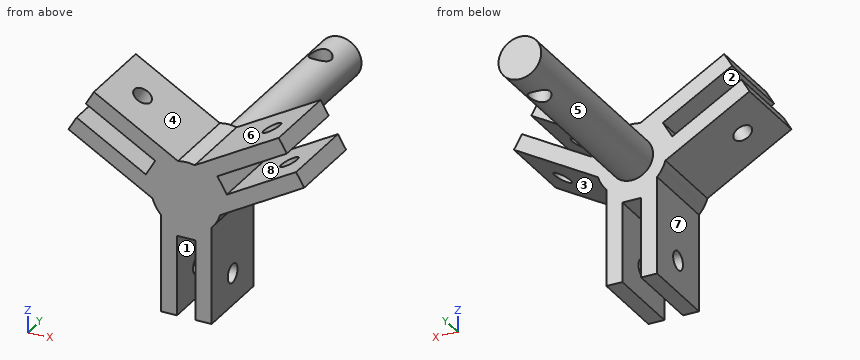
```python
from build123d import *

# Parameters (mm, degrees)
EXTRUDE_1_DEPTH     = 15
SKETCH_2_R          = 4
EXTRUDE_2_DEPTH     = 40
SKETCH_3_R          = 1.75
CUT_EXTRUDE_1_DEPTH = 15
SKETCH_4_R          = 1.75
CUT_EXTRUDE_2_DEPTH = 15
SKETCH_5_R          = 1.75
CUT_EXTRUDE_3_DEPTH = 15
SKETCH_7_R          = 2
CUT_EXTRUDE_4_DEPTH = 15


with BuildPart() as part:
    # 草圖1 → 填料-伸長1 (new body)
    with BuildSketch(Plane(origin=(0, 0, 0), x_dir=(1, 0, 0), z_dir=(0, 1, 0))):
        with BuildLine():
            Line((6.314953067, 1.838887704), (22.070508076, -7.257586221))
            Line((22.070508076, -7.257586221), (20.570508076, -9.855662433))
            Line((20.570508076, -9.855662433), (7.580127019, -2.355662433))
            Line((7.580127019, -2.355662433), (5.830127019, -5.386751346))
            Line((5.830127019, -5.386751346), (18.820508076, -12.886751346))
            Line((18.820508076, -12.886751346), (17.320508076, -15.484827557))
            Line((17.320508076, -15.484827557), (1.564953067, -6.388353632))
            ThreePointArc((1.564953067, -6.388353632), (0, -6.577244121), (-1.564953067, -6.388353632))
            Line((-1.564953067, -6.388353632), (-17.320508076, -15.484827557))
            Line((-17.320508076, -15.484827557), (-18.820508076, -12.886751346))
            Line((-18.820508076, -12.886751346), (-5.830127019, -5.386751346))
            Line((-5.830127019, -5.386751346), (-7.580127019, -2.355662433))
            Line((-7.580127019, -2.355662433), (-20.570508076, -9.855662433))
            Line((-20.570508076, -9.855662433), (-22.070508076, -7.257586221))
            Line((-22.070508076, -7.257586221), (-6.314953067, 1.838887704))
            ThreePointArc((-6.314953067, 1.838887704), (-5.696060496, 3.28862206), (-4.75, 4.549465928))
            Line((-4.75, 4.549465928), (-4.75, 22.742413779))
            Line((-4.75, 22.742413779), (-1.75, 22.742413779))
            Line((-1.75, 22.742413779), (-1.75, 7.742413779))
            Line((-1.75, 7.742413779), (1.75, 7.742413779))
            Line((1.75, 7.742413779), (1.75, 22.742413779))
            Line((1.75, 22.742413779), (4.75, 22.742413779))
            Line((4.75, 22.742413779), (4.75, 4.549465928))
            ThreePointArc((4.75, 4.549465928), (5.696060496, 3.28862206), (6.314953067, 1.838887704))
        make_face()
    extrude(amount=EXTRUDE_1_DEPTH)

    # 草圖2 → 填料-伸長2 (add)
    with BuildSketch(Plane(origin=(0, 15, 0), x_dir=(1, 0, 0), z_dir=(0, 1, 0))):
        Circle(SKETCH_2_R)
    extrude(amount=EXTRUDE_2_DEPTH)

    # 草圖3 → 除料-伸長1 (cut)
    with BuildSketch(Plane(origin=(4.75, 0, 0), x_dir=(0, 0, -1), z_dir=(1, 0, 0))):
        with Locations((16.742413779, 7.5)):
            Circle(SKETCH_3_R)
    extrude(amount=-CUT_EXTRUDE_1_DEPTH, mode=Mode.SUBTRACT)

    # 草圖4 → 除料-伸長2 (cut)
    with BuildSketch(Plane(origin=(-2.375, 0, -4.113620668), x_dir=(-0.866025404, 0, 0.5), z_dir=(-0.5, 0, -0.866025404))):
        with Locations((16.742413779, 7.5)):
            Circle(SKETCH_4_R)
    extrude(amount=-CUT_EXTRUDE_2_DEPTH, mode=Mode.SUBTRACT)

    # 草圖5 → 除料-伸長3 (cut)
    with BuildSketch(Plane(origin=(-2.375, 0, 4.113620668), x_dir=(0.866025404, 0, 0.5), z_dir=(-0.5, 0, 0.866025404))):
        with Locations((16.742413779, 7.5)):
            Circle(SKETCH_5_R)
    extrude(amount=-CUT_EXTRUDE_3_DEPTH, mode=Mode.SUBTRACT)

    # 草圖7 → 除料-伸長4 (cut)
    with BuildSketch(Plane.XY.offset(4)):
        with Locations((0, 48)):
            Circle(SKETCH_7_R)
    extrude(amount=-CUT_EXTRUDE_4_DEPTH, mode=Mode.SUBTRACT)


solid = part.part
```
Source: CAD feature listing. Evaluate the final solid. Frame: model axes, mm. Face numbers are marked on the shaded views. A direction names the side the tool comes from. Coordinates: 2 decimals unless noted, no trailing zeros. Loops run counter-clockwise (first coordinate to the right, second up) from the corner with the lowest first, then second, coordinate; pieces in that order, holes last. Notation, with made-up numbers: M 80.5,64 L 129.5,64 A27 cw 129.5,94 Z; hole C 76,43 d6. An arc over 180 degrees is marked long. Use CSV: the item, a comma, the result in double quotes.
(1) Cut plane D-D on z = 0. Return loops of the section in (x, y), and give its area (3 significant figures).
Answers follow:
outline,"M -9.5,0 L 9.5,0 L 9.5,15 L 4,15 L 4,55 L -4,55 L -4,15 L -9.5,15 Z; hole C 0,48 d4"
area,"592 mm²"
(2) Line query: line 1 (X direction, y = 14, z = 5.5); line 2 (X direction, y = 14, z = -15); line 3 (Y direction, x = 0, z = -2). Output: solid intervals per line, ascending. Write a range as [from, to].
Answers follow:
line 1,"[-19.03, -13.03], [-6.03, 6.03], [13.03, 19.03]"
line 2,"[-4.75, -1.75], [1.75, 4.75]"
line 3,"[0, 46], [50, 55]"
(3) Reachability of the marked faces 5, 6, 7 and 8 from +Z, -Z, +X, -X, +Y, -Y: full face, straight path, thin tool, end or side. Return the list, or none.
Answers follow:
face 5,"+Y"
face 6,"+Z, +Y, -Y"
face 7,"-Z, -X, +Y, -Y"
face 8,"+Y, -Y"
(4) Contact query for flat-ended pins moving along their axis: pin 1 (3 mm diameter, centred on y = 41.5, z = -4, fed in from -X); pin 2 (7.5 mm diameter, centred on y = 10.5, z = -17, fed in from -X); pin 3 (7.5 mm diameter, centred on y = 9, z = -17, fed in from +X). Output: stop coordinate, or through.
Answers follow:
pin 1,"x = -3.12"
pin 2,"x = -4.75"
pin 3,"x = 4.75"
(5) Cut plane C-C on y = 14. Return loops of the section in (x, z), and give its area (3 significant figures).
Answers follow:
outline,"M -22.07,7.26 L -6.31,-1.84 A6.58 ccw -4.75,-4.55 L -4.75,-22.74 L -1.75,-22.74 L -1.75,-7.74 L 1.75,-7.74 L 1.75,-22.74 L 4.75,-22.74 L 4.75,-4.55 A6.58 ccw 6.31,-1.84 L 22.07,7.26 L 20.57,9.86 L 7.58,2.36 L 5.83,5.39 L 18.82,12.89 L 17.32,15.48 L 1.56,6.39 A6.58 ccw -1.56,6.39 L -17.32,15.48 L -18.82,12.89 L -5.83,5.39 L -7.58,2.36 L -20.57,9.86 Z"
area,"457 mm²"
(6) Draft query along Z for the marked faces 1, 2, 3 and 4. Return one class per face: pulls with the +Z half, pulls with the -Z half, needs draft (parallel to the pull), parting line crosses it, or undercut.
Answers follow:
face 1,"needs draft"
face 2,"undercut"
face 3,"pulls with the -Z half"
face 4,"pulls with the +Z half"
(7) Cut plane A-A on z = -12. Return loops of the section in (x, y), and give its area (3 significant figures).
Answers follow:
outline,"M -4.75,0 L -1.75,0 L -1.75,15 L -4.75,15 Z; M 1.75,0 L 4.75,0 L 4.75,15 L 1.75,15 Z"
area,"90.0 mm²"
(8) Cut plane B-B on x = 0. Return loops of the section in (y, z).
Answers follow:
outline,"M 0,-7.74 L 15,-7.74 L 15,-4 L 46,-4 L 46,4 L 15,4 L 15,6.58 L 0,6.58 Z; M 50,-4 L 55,-4 L 55,4 L 50,4 Z"
